The figure shows three views and two pictorial views of one solid part (mm, origin at its lowest corner). Answer the questions. Coordinates: 2 decimals unless noted, no trailing zeros. Order: outer loops, then holes, each group sorted by start corner. A loop starts at its lowest first (then second) coordinate and runs counter-clockwise, first axis right, second up. Notation, with made-up numbers: M -13.5,-15 L 14.5,-15 A19 cw 14.5,-9 Z; hole C 86,-5.5 d6. An arc over 180 degrees is marked long. Answer in a Markdown table with one row per item. Add a question column.
Item 1: Consider line 1 (Z direction, x = 8.5, y = 25) (3 decimals); line 2 (X direction, y = 29, z = 55). Determine where each line is inside the solid, lowest interval first. Write a range as from..to.
Item 2: Flat-ended cylindrical pins translate along their axes: pin 1 Ø5 at (y, z) = (17, 4.5) entering from +X; pin 2 Ø1.5 at (x, y) = (8.5, 23) entering from +Z (3 decimals); pin 3 Ø12 at (y, z) = (3.5, 141.5) entering from -X; pin 4 Ø1.6 at (x, y) = (8, 20.5) entering from -Z (3 decimals). Find the tip coordinate at first contact, or state that the pin passes through.
Item 3: The part is cut by section A-A (y = 18). Write down the section's boundary in (x, z) (3 decimals).
Item 4: The part is cut by section B-B (z = 59). Write down the section's boundary in (x, y), then the cut area to 3 significant figures.
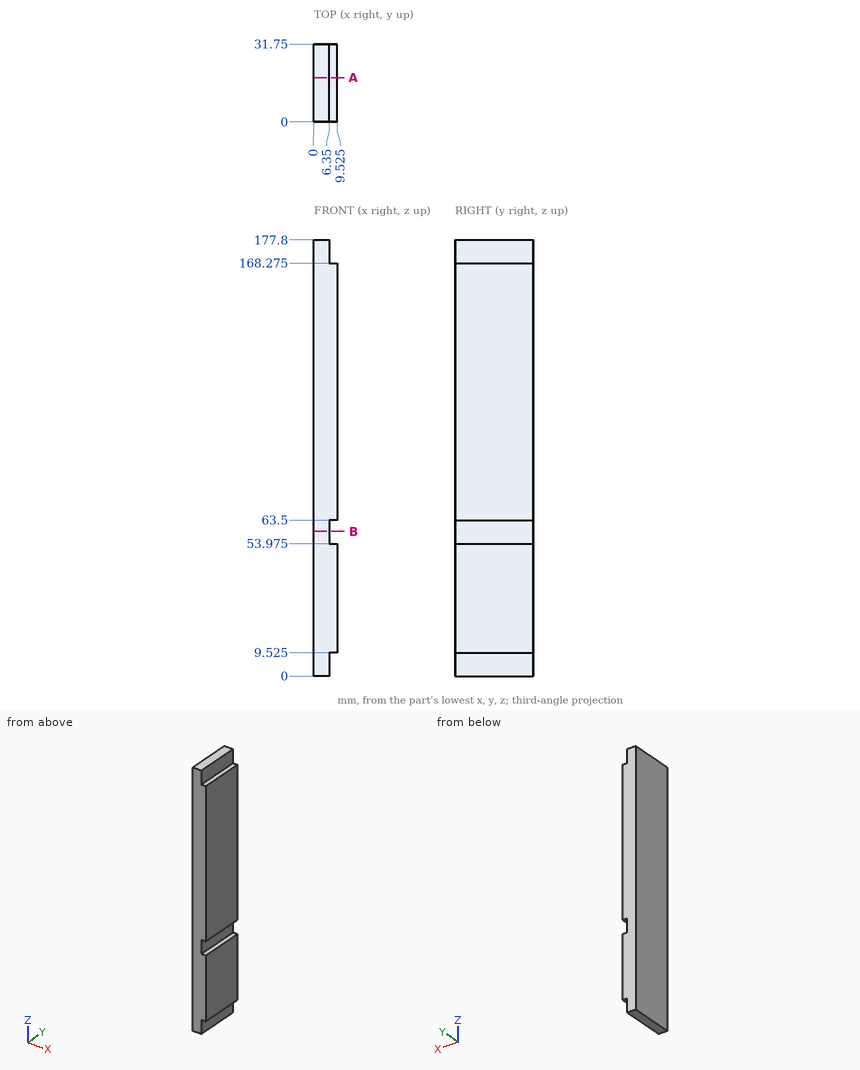
Reply:
| question | item | result |
|---|---|---|
| 1 | line 1 | z = 9.525..53.975, 63.5..168.275 |
| 1 | line 2 | x = 0..6.35 |
| 2 | pin 1 | stops at x = 6.35 |
| 2 | pin 2 | stops at z = 168.275 |
| 2 | pin 3 | stops at x = 0 |
| 2 | pin 4 | stops at z = 9.525 |
| 3 | outline | M 0,0 L 6.35,0 L 6.35,9.525 L 9.525,9.525 L 9.525,53.975 L 6.35,53.975 L 6.35,63.5 L 9.525,63.5 L 9.525,168.275 L 6.35,168.275 L 6.35,177.8 L 0,177.8 Z |
| 4 | outline | M 0,0 L 6.35,0 L 6.35,31.75 L 0,31.75 Z |
| 4 | area | 202 mm2 |
